The listing builds one solid part. Answer for the finished solid, in the listing's coordinates (mm). A direction names the side the tool comes from. Coordinates: 2 decimals unless noted, no trailing zeros. Loops run counter-clockwise (first coordinate to the right, second up) from the corner with the lowest first, then second, coordinate; pieces in that order, holes last. Notation, with made-up numbers: (59, 63) -> (96, 63) arc R16 ccw to (96, 67) -> close; hole circle Ø9 at (-27.75, 89.5). An arc over 180 degrees is marked (long way). Answer in a Markdown table with one row per item.
```python
from build123d import *

# Parameters (mm, degrees)
F0_W     = 12.14
F0_H     = 24.3
F1_DEPTH = 10
F2_R     = 2.5
F3_DEPTH = 1.1
F4_R     = 2
F5_DEPTH = 0.7
F7_DEPTH = 5


with BuildPart() as f1:
    # F0 (on Top) → F1 (new body)
    with BuildSketch(Plane.XY):
        with Locations((-49.791635, 32.747907)):
            Rectangle(F0_W, F0_H)
    extrude(amount=F1_DEPTH)

    # F2 (on face) → F3 (join)
    with BuildSketch(Plane(origin=(0, 44.897907, 0), x_dir=(-1, 0, 0), z_dir=(0, 1, 0))):
        with Locations((49.791635, 5)):
            Circle(F2_R)
    extrude(amount=F3_DEPTH)

    # F4 (on face) → F5 (join)
    with BuildSketch(Plane.XZ.offset(-20.597907)):
        with Locations((-49.791635, 5)):
            Circle(F4_R)
    extrude(amount=F5_DEPTH)

    # F6 (on face) → F7 (join)
    with BuildSketch(Plane.XZ.offset(-19.897907)):
        with BuildLine():
            ThreePointArc((-50.931811, 6.05), (-50.355208, 3.556087), (-48.241635, 5))
            ThreePointArc((-48.241635, 5), (-48.347722, 5.563573), (-48.65146, 6.05))
            Line((-48.65146, 6.05), (-50.931811, 6.05))
        make_face()
    extrude(amount=F7_DEPTH)


with BuildPart() as f8_1:
    # F8: copy of F1
    add(f1.part.moved(Location((20, 0, 0))))


solid = f1.part
```
Item 1: A cutting plane is placed at D-D, the plane x = -53.5. Determine the outline of the cut face in (y, z).
Findings below:
| item | result |
|---|---|
| outline | (20.6, 0) -> (44.9, 0) -> (44.9, 10) -> (20.6, 10) -> close |
Item 2: A cutting plane is placed at A-A, the plane z = 3.75. Determine the outline of the cut face in (x, y), plus the area to 3 significant figures.
Findings below:
| item | result |
|---|---|
| outline | (-55.86, 20.6) -> (-51.35, 20.6) -> (-51.35, 19.9) -> (-50.71, 19.9) -> (-50.71, 14.9) -> (-48.88, 14.9) -> (-48.88, 19.9) -> (-48.23, 19.9) -> (-48.23, 20.6) -> (-43.72, 20.6) -> (-43.72, 44.9) -> (-47.63, 44.9) -> (-47.63, 46) -> (-51.96, 46) -> (-51.96, 44.9) -> (-55.86, 44.9) -> close |
| area | 311 mm2 |
Item 3: Flat-ended cylindrical pins translate along their axes: pin 1 Ø3 at (x, z) = (-50.5, 8.5) entering from -Y; pin 2 Ø2.5 at (x, y) = (-49.5, 18.5) entering from +Z; pin 3 Ø6 at (x, z) = (-46.5, 4) entering from -Y. Find the tip coordinate at first contact, or state that the pin passes through.
Findings below:
| item | result |
|---|---|
| pin 1 | stops at y = 20.6 |
| pin 2 | stops at z = 6.05 |
| pin 3 | stops at y = 14.9 |
Item 4: A tool of negligible diameter and unlimited length cuts with its end or side. For faces 1 (the face through (-49.8, 19.898, 6.4)), 2 (the face through (-50, 45.998, 5)), 3 (the face through (-52.176, 45.44, 5.751)), 4 (the face through (-50, 17, 6.05)), from which of +Z, -Z, +X, -X, +Y, -Y can it reach the whole face along a straight path? Write none if from no direction.
Findings below:
| item | result |
|---|---|
| face 1 | -Y |
| face 2 | +Z, -Z, +X, -X, +Y |
| face 3 | +Y |
| face 4 | +Z, +X, -X, -Y |
Item 5: A cutting plane is placed at C-C, the plane y = 17.5. Determine the outline of the cut face in (x, z), plus the area to 3 significant figures.
Findings below:
| item | result |
|---|---|
| outline | (-50.93, 6.05) arc R1.55 ccw (long way) to (-48.24, 5) arc R1.55 ccw to (-48.65, 6.05) -> close |
| area | 6.76 mm2 |
Item 6: A cutting plane is placed at B-B, the plane x = -49.5. Determine the outline of the cut face in (y, z).
Findings below:
| item | result |
|---|---|
| outline | (14.9, 3.48) -> (19.9, 3.48) -> (19.9, 3.02) -> (20.6, 3.02) -> (20.6, 0) -> (44.9, 0) -> (44.9, 2.52) -> (46, 2.52) -> (46, 7.48) -> (44.9, 7.48) -> (44.9, 10) -> (20.6, 10) -> (20.6, 6.98) -> (19.9, 6.98) -> (19.9, 6.05) -> (14.9, 6.05) -> close |
Item 7: Find the intervals of material crossed by probe 1 along Y at (x, z) = (-44.5, 3); probe 2 along Y at (x, z) = (-50, 6.5); probe 3 along Z at (x, y) = (-48.5, 18.5), in increasing order.
Findings below:
| item | result |
|---|---|
| probe 1 | y = 20.6 to 44.9 |
| probe 2 | y = 19.9 to 46 |
| probe 3 | z = 4.14 to 5.86 |
